Input: part model. Units: mm. Frame: model coordinates. A direction names the side the tool comes from. Give positions to 0.01 mm unless a question says otherwise; leave off trailing zeros. Write each loop counter-clockwise with the first axis right and the second up, starting at its lowest first coordinate (ties: lowest second). Pieces come first, ordered by that corner, then holes. Notation, with made-up numbers: (82, 70) -> (119, 70) arc R15 ccw to (119, 96) -> close; hole circle Ø11 at (-7.5, 5.5). An arc over 180 degrees is marked (long way). Answer as a JSON object with one key per item and string values. Group by question number.
from build123d import *

# Parameters (mm, degrees)
BOSS_EXTRUDE1_DEPTH  = 12.5
M5_CLEARANCE_HOLE1_D = 5.3
SKETCH4_W            = 1
SKETCH4_H            = 20
CUT_EXTRUDE1_DEPTH   = 3


with BuildPart() as part:
    # Sketch1 → Boss-Extrude1 (new body, symmetric)
    with BuildSketch(Plane.XY):
        with BuildLine():
            Line((-15.2, 0), (-12.7, 0))
            ThreePointArc((-12.7, 0), (0, 12.7), (12.7, 0))
            Line((12.7, 0), (15.2, 0))
            Line((15.2, 0), (15.2, 5.2))
            ThreePointArc((15.2, 5.2), (12.271067812, 12.271067812), (5.2, 15.2))
            Line((5.2, 15.2), (-5.2, 15.2))
            ThreePointArc((-5.2, 15.2), (-12.271067812, 12.271067812), (-15.2, 5.2))
            Line((-15.2, 5.2), (-15.2, 0))
        make_face()
    extrude(amount=BOSS_EXTRUDE1_DEPTH, both=True)

    # M5 Clearance Hole1 (through all)
    with Locations(Plane(origin=(0, 15.2, 0), x_dir=(1, 0, 0), z_dir=(0, 1, 0))):
        with Locations((0, 0)):
            Hole(M5_CLEARANCE_HOLE1_D / 2)

    # Sketch4 → Cut-Extrude1 (cut)
    with BuildSketch(Plane.XZ):
        with Locations((-13.95, 0)):
            Rectangle(SKETCH4_W, SKETCH4_H)
        with Locations((13.95, 0)):
            Rectangle(SKETCH4_W, SKETCH4_H)
    extrude(amount=-CUT_EXTRUDE1_DEPTH, mode=Mode.SUBTRACT)


solid = part.part
1. Section A-A (x = 0). Return the cut outline in (y, z), plus the area to 4 significant figures.
2. Reachability of faces 1 (the face through (-15, 0, 0)), 2 (the face through (13.45, 1, 0)) from +Z, -Z, +X, -X, +Y, -Y: full face, straight path, thin tool, end or side. Return the list, or none.
3. Contact query for flat-ended pins moving along their axis: pin 1 Ø4 at (x, y) = (-9.5, 2) entering from -Z; pin 2 Ø4 at (x, z) = (10, -1.5) entering from +Y; pin 3 Ø0.8 at (x, z) = (14, -3) entering from -Y. Output: stop coordinate, or through.
4. Section C-C (y = 1.75). Return the cut outline in (x, z), plus the area to 3 significant figures.
5. Mould query, pull axis Z, two halves, no side actions, for faces 3 (the face through (-13.45, 1, 0)), 4 (the face through (0, 13, -12.5)), 5 (the face through (14.45, 1, 0)), 6 (the face through (-12.19, 12.35, 0.18)). Classes: pulls with the +Z half, pulls with the -Z half, needs draft (parallel to the pull), parting line crosses it, or undercut.
6. Section D-D (y = 12). Return the cut outline in (x, z).
7. Section B-B (z = 0). Return the cut outline in (x, y).
8. Line query: line 1 (Z direction, x = 0, y = 14.2); line 2 (X direction, y = 1, z = -8.25); line 3 (X direction, y = 6, z = -2). Output: solid intervals per line, ascending.
Working result:
{
 "1": {"outline": "(12.7, -12.5) -> (15.2, -12.5) -> (15.2, -2.65) -> (12.7, -2.65) -> close; (12.7, 2.65) -> (15.2, 2.65) -> (15.2, 12.5) -> (12.7, 12.5) -> close", "area": "49.25 mm^2"},
 "2": {"face 1": "+Z, -Z, +X, -X, -Y", "face 2": "-Y"},
 "3": {"pin 1": "passes through", "pin 2": "stops at y = 14.8", "pin 3": "stops at y = 3"},
 "4": {"outline": "(-15.2, -12.5) -> (-12.58, -12.5) -> (-12.58, 12.5) -> (-15.2, 12.5) -> close; (12.58, -12.5) -> (15.2, -12.5) -> (15.2, 12.5) -> (12.58, 12.5) -> close; hole (-14.45, -10) -> (-13.45, -10) -> (-13.45, 10) -> (-14.45, 10) -> close; hole (13.45, -10) -> (14.45, -10) -> (14.45, 10) -> (13.45, 10) -> close", "area": "91.1 mm^2"},
 "5": {"face 3": "undercut", "face 4": "pulls with the -Z half", "face 5": "undercut", "face 6": "needs draft"},
 "6": {"outline": "(-12.53, -12.5) -> (-4.16, -12.5) -> (-4.16, 12.5) -> (-12.53, 12.5) -> close; (4.16, -12.5) -> (12.53, -12.5) -> (12.53, 12.5) -> (4.16, 12.5) -> close"},
 "7": {"outline": "(-15.2, 0) -> (-14.45, 0) -> (-14.45, 3) -> (-13.45, 3) -> (-13.45, 0) -> (-12.7, 0) arc R12.7 cw to (-2.65, 12.42) -> (-2.65, 15.2) -> (-5.2, 15.2) arc R10 ccw to (-15.2, 5.2) -> close; (2.65, 12.42) arc R12.7 cw to (12.7, 0) -> (13.45, 0) -> (13.45, 3) -> (14.45, 3) -> (14.45, 0) -> (15.2, 0) -> (15.2, 5.2) arc R10 ccw to (5.2, 15.2) -> (2.65, 15.2) -> close"},
 "8": {"line 1": "z = -12.5 to -2.65, 2.65 to 12.5", "line 2": "x = -15.2 to -14.45, -13.45 to -12.66, 12.66 to 13.45, 14.45 to 15.2", "line 3": "x = -15.17 to -11.19, 11.19 to 15.17"}
}
